```python
from build123d import *

# Parameters (mm, degrees)
F0_R     = 12.7
F1_DEPTH = 6.35


with BuildPart() as f1:
    # F0 (on Top) → F1 (new body)
    with BuildSketch(Plane.XY):
        with BuildLine():
            Line((-46.93308, 19.440318), (-58.66635, 24.300398))
            ThreePointArc((-58.66635, 24.300398), (-62.279865, 12.388235), (-63.5, 0))
            Line((-63.5, 0), (-50.8, 0))
            ThreePointArc((-50.8, 0), (-50.08849, -8.472496), (-47.97389, -16.707658))
            Line((-47.97389, -16.707658), (-59.72273, -21.574187))
            ThreePointArc((-59.72273, -21.574187), (-53.596494, -34.053866), (-44.901281, -44.901281))
            Line((-44.901281, -44.901281), (-35.921024, -35.921024))
            ThreePointArc((-35.921024, -35.921024), (-28.222968, -42.238656), (-19.440318, -46.93308))
            Line((-19.440318, -46.93308), (-24.300398, -58.66635))
            ThreePointArc((-24.300398, -58.66635), (-12.388235, -62.279865), (0, -63.5))
            Line((0, -63.5), (0, -50.8))
            ThreePointArc((0, -50.8), (9.910588, -49.823892), (19.440318, -46.93308))
            Line((19.440318, -46.93308), (24.300398, -58.66635))
            ThreePointArc((24.300398, -58.66635), (35.27871, -52.79832), (44.901281, -44.901281))
            Line((44.901281, -44.901281), (35.921024, -35.921024))
            ThreePointArc((35.921024, -35.921024), (42.238656, -28.222968), (46.93308, -19.440318))
            Line((46.93308, -19.440318), (58.66635, -24.300398))
            ThreePointArc((58.66635, -24.300398), (62.279865, -12.388235), (63.5, 0))
            Line((63.5, 0), (50.8, 0))
            ThreePointArc((50.8, 0), (49.823892, 9.910588), (46.93308, 19.440318))
            Line((46.93308, 19.440318), (58.66635, 24.300398))
            ThreePointArc((58.66635, 24.300398), (52.79832, 35.27871), (44.901281, 44.901281))
            Line((44.901281, 44.901281), (35.921024, 35.921024))
            ThreePointArc((35.921024, 35.921024), (28.222968, 42.238656), (19.440318, 46.93308))
            Line((19.440318, 46.93308), (24.300398, 58.66635))
            ThreePointArc((24.300398, 58.66635), (12.388235, 62.279865), (0, 63.5))
            Line((0, 63.5), (0, 50.8))
            ThreePointArc((0, 50.8), (-9.910588, 49.823892), (-19.440318, 46.93308))
            Line((-19.440318, 46.93308), (-24.300398, 58.66635))
            ThreePointArc((-24.300398, 58.66635), (-35.27871, 52.79832), (-44.901281, 44.901281))
            Line((-44.901281, 44.901281), (-35.921024, 35.921024))
            ThreePointArc((-35.921024, 35.921024), (-42.238656, 28.222968), (-46.93308, 19.440318))
        make_face()
        Circle(F0_R, mode=Mode.SUBTRACT)
    extrude(amount=F1_DEPTH)


solid = f1.part
```
Source: CAD feature listing. Evaluate the final solid. Frame: model axes, mm. A direction names the side the tool comes from. Give positions to 0.01 mm unless a question says otherwise; leave off trailing zeros. Loops run counter-clockwise (first coordinate to the right, second up) from the corner with the lowest first, then second, coordinate; pieces in that order, holes last. Notation, with made-up numbers: (-19.5, 88.5) - (21.5, 88.5) arc R15 ccw to (21.5, 117.5) - close; hole circle Ø5 at (65, 69). An arc over 180 degrees is marked (long way). Use CSV: the item, a comma, the result in double quotes. Start each with the question number.
1. Reachability of faces 5 (the flat face through (-21.836, 52.718, 3.131)), 6 (the flat face through (52.718, -21.836, 3.131)), 7 (the flat face through (-21.836, -52.718, 3.131)), 8 (the cylindrical face through (-42.16, 28.34, 3.13)) from +Z, -Z, +X, -X, +Y, -Y: full face, straight path, thin tool, end or side. Return the list, or none.
2. Pin query (flat end, axial travel): pin 1 (2 mm diameter, centred on x = 22.5, z = 2.5, fed in from +Y); pin 2 (1.9 mm diameter, centred on x = 55, z = 4.5, fed in from +Y); pin 3 (2 mm diameter, centred on y = -11.5, z = 4, fed in from +X). Return the tip coordinate at first contact, or that it passes through.
3. Section A-A (x = 48.5). Output: boundary loops of the cut face in (y, z), then the cut area to 3 significant figures.
4. Section D-D (x = 28). Output: boundary loops of the cut face in (y, z).
5. Ray query, L1, parallel to X at y = -10, z = 3; L2, parallel to X at y = 23.5, z = 3.75; L3, parallel to Y at x = 42, z = 5.25. Return the intervals inside material, ascending.
6. Draft query along Y for faces 1 (the flat face through (-40, 40, 3)), 2 (the cylindrical face through (42.16, -28.34, 3.13)), 3 (the cylindrical face through (9.77, -49.85, 3.13)), 4 (the flat face through (-52.718, 21.836, 3.131)). Return one class per face: +Y half, -Y half, draft (parallel to the pull), parting line (faces both ways), or undercut.
7. Section C-C (y = 21.5). Output: boundary loops of the cut face in (x, z), then the cut area to 3 significant figures.
Response:
1,face 5,"+Z, -Z, +Y"
1,face 6,"+Z, -Z, -Y"
1,face 7,"+Z, -Z, -X"
1,face 8,"+Z, -Z"
2,pin 1,"y = 59.75"
2,pin 2,"y = 33.33"
2,pin 3,"x = 62.63"
3,outline,"(-20.09, 0) - (15.11, 0) - (15.11, 6.35) - (-20.09, 6.35) - close; (20.09, 0) - (40.99, 0) - (40.99, 6.35) - (20.09, 6.35) - close"
3,area,"356 mm²"
4,outline,"(-56.99, 0) - (42.39, 0) - (42.39, 6.35) - (-56.99, 6.35) - close"
5,L1,"-49.81 to -7.83, 7.83 to 62.71"
5,L2,"-58.99 to -56.73, -45.04 to 56.73"
5,L3,"-47.63 to -42, -28.58 to 42"
6,face 1,"undercut"
6,face 2,"undercut"
6,face 3,"-Y half"
6,face 4,"+Y half"
7,outline,"(-59.75, 0) - (-51.91, 0) - (-51.91, 6.35) - (-59.75, 6.35) - close; (-46.03, 0) - (51.91, 0) - (51.91, 6.35) - (-46.03, 6.35) - close"
7,area,"672 mm²"
